Input: part model. Units: mm. Frame: model coordinates. A direction names the side the tool comes from. Coordinates: 2 decimals unless noted, no trailing zeros. Loops run counter-clockwise (first coordinate to the right, second up) from the corner with the lowest first, then second, coordinate; pieces in that order, holes last.
Item 1: Section D-D on x = -87.5. Return loops of the section in (y, z).
Item 2: Section B-B on y = -7.5. Return loops of the section in (x, z).
Item 3: Section A-A on x = 23.5. Return loops of the section in (y, z).
Item 4: Ray query, line 1 along X through (y, z) = (-76, 96.5); line 2 along X through (y, z) = (-56.5, 39); line 3 along Y through (x, z) = (-25, 22.5). Return the intervals inside material, ascending.
Item 5: Reachability of faces 1 (the flat face through (100, -27.5, 2)), 2 (the flat face through (27.5, -100, 2)), 3 (the flat face through (125, -62, 2)), 4 (the flat face through (-23, -27.5, 2)), 5 (the flat face through (110, 110, 2)) from +Z, -Z, +X, -X, +Y, -Y: full face, straight path, thin tool, end or side. Return the list, or none.
Item 6: Section C-C on z = 12. Return loops of the section in (x, y).
Item 7: Pull-direction query (Y, two-part tool) for faces 6 (the flat face through (0, -75, 2)), 7 (the flat face through (-30, 30, -125)), 8 (the flat face through (0, 75, 2)), 9 (the flat face through (-110, 110, 2)); classes: released by +Y, released by -Y, zero draft, split by the parting line, or undercut.
```python
from build123d import *

# Parameters (mm, degrees)
F0_R     = 20
F1_DEPTH = 125


with BuildPart() as f1:
    # F0 (on Top) → F1 (new body, symmetric)
    with BuildSketch(Plane.XY):
        Polygon((27.5, -125), (95, -125), (125, -95), (125, -27.5), (75, -27.5), (75, 27.5), (125, 27.5), (125, 95), (95, 125), (-95, 125), (-125, 95), (-125, -95), (-95, -125), (-27.5, -125), (-27.5, -75), (27.5, -75), align=None)
        with Locations((-75, -75)):
            Circle(F0_R, mode=Mode.SUBTRACT)
        with Locations((75, -75)):
            Circle(F0_R, mode=Mode.SUBTRACT)
        Polygon((27.5, -27.5), (-75, -27.5), (-75, 27.5), (-27.5, 27.5), (-27.5, 75), (27.5, 75), align=None, mode=Mode.SUBTRACT)
        with Locations((-75, 75)):
            Circle(F0_R, mode=Mode.SUBTRACT)
        with Locations((75, 75)):
            Circle(F0_R, mode=Mode.SUBTRACT)
    extrude(amount=F1_DEPTH, both=True)


solid = f1.part
```
Results found:
1. outline: (-125, -125) - (-90.61, -125) - (-90.61, 125) - (-125, 125) - close; (-59.39, -125) - (59.39, -125) - (59.39, 125) - (-59.39, 125) - close; (90.61, -125) - (125, -125) - (125, 125) - (90.61, 125) - close
2. outline: (-125, -125) - (-75, -125) - (-75, 125) - (-125, 125) - close; (27.5, -125) - (75, -125) - (75, 125) - (27.5, 125) - close
3. outline: (-75, -125) - (-27.5, -125) - (-27.5, 125) - (-75, 125) - close; (75, -125) - (125, -125) - (125, 125) - (75, 125) - close
4. line 1: x = -125 to -94.97, -55.03 to -27.5, 27.5 to 55.03, 94.97 to 125
4. line 2: x = -125 to -82.6, -67.4 to 67.4, 82.6 to 125
4. line 3: y = -75 to -27.5, 75 to 125
5. face 1: +Z, -Z, +X
5. face 2: +Z, -Z, -Y
5. face 3: +Z, -Z, +X, +Y, -Y
5. face 4: +Z, -Z
5. face 5: +Z, -Z, +X, +Y
6. outline: (-125, -95) - (-95, -125) - (-27.5, -125) - (-27.5, -75) - (27.5, -75) - (27.5, -125) - (95, -125) - (125, -95) - (125, -27.5) - (75, -27.5) - (75, 27.5) - (125, 27.5) - (125, 95) - (95, 125) - (-95, 125) - (-125, 95) - close; hole circle Ø40 at (-75, -75); hole circle Ø40 at (-75, 75); hole (-75, -27.5) - (27.5, -27.5) - (27.5, 75) - (-27.5, 75) - (-27.5, 27.5) - (-75, 27.5) - close; hole circle Ø40 at (75, -75); hole circle Ø40 at (75, 75)
7. face 6: released by -Y
7. face 7: zero draft
7. face 8: undercut
7. face 9: released by +Y
